Autodesk Fusion 360 part; units mm, degrees
sketch "Sketch1" plane through (0, 0, 0) normal (0, 1, 0) x (1, 0, 0) in component "Oil Drop Cap"
  circle A0 centre (0, 0) radius 6.2
  circle A1 centre (0, 0) radius 1.45
  dimension "d5" = 12.4
  dimension "d6" = 2.9
sketch "Sketch2" plane through (0, 0, 0) normal (1, 0, 0) x (0, 0, -1) in component "Oil Drop Cap"
  line L0 (0, 0) -> (0, 3.8) construction
  circle A0 centre (0, 3.8) radius 1.45
  dimension "d7" = 3.8
  dimension "d8" = 2.9
extrude "Extrude1" add sketch "Sketch1" along normal blind 10.3 contours A0 | A1 in component "Oil Drop Cap"
extrude "Extrude2" cut sketch "Sketch2" along normal up to surface end surface at (6.1923, 6.8667, 0.309) in component "Oil Drop Cap"
extrude "Extrude3" cut sketch "Sketch1" along normal up to surface contours A1 end surface at (2.0667, 5.25, 0) in component "Oil Drop Cap"
chamfer "Chamfer1" distance 0.25 angle 45 2 faces at (1.6068, 10.3, -0.7965) (4.5882, 0, 0.3801) in component "Oil Drop Cap"
chamfer "Chamfer1" distance 0.25 angle 45 1 edges at (6.0281, 3.8, 1.45) in component "Oil Drop Cap"
component "Oil Drop Cap" placed x (1, 0, 0) y (0, 1, 0) z (0, 0, 1) at (0, 0, 0)
equation "CylinderDiameter = 12.4 mm"
equation "CylinderHeight = 10.3 mm"
equation "HoleDiameter = 2.9 mm"
equation "HoleHeight = 3.8 mm"
equation "d5 = CylinderDiameter"
equation "d6 = HoleDiameter"
equation "d7 = HoleHeight"
equation "d8 = HoleDiameter"
equation "d9 = CylinderHeight"
CAD build for the part. Positions are in the model's coordinates, mm. A direction names the side the tool comes from. Round coordinates to 2 decimals unless told otherwise and drop trailing zeros. Order: outer loops, then holes, each group sorted by start corner. A loop starts at its lowest first (then second) coordinate and runs counter-clockwise, first axis right, second up. Notation, with made-up numbers: (-39, 76.25) - (-18, 76.25) arc R20 cw to (-18, 82.25) - close; hole circle Ø8 at (-17.5, 17). An arc over 180 degrees is marked (long way). Answer as CSV lines item,"result". Start each with the question number.
1. Pin check, flat tips, straight feed: pin 1 (2.5 mm diameter, centred on x = 0, z = 0, fed in from -Y); pin 2 (5 mm diameter, centred on y = 4, z = 2.5, fed in from +X); pin 3 (1 mm diameter, centred on y = 4, z = -1.5, fed in from -X). Stop position of each tip, or through.
2. Pull direction Z, two halves, no side cores. Call faces 1 (the face through (-0.57, 2.35, -0.03)), 2 (the face through (0, 10.3, 0)), 3 (the face through (2.86, 5.08, -5.5)): +Z half, -Z half, draft (parallel to the pull), parting line (faces both ways), or undercut.
3. Saw through at A-A, the plane y = 9. Write the cut outline in (x, z).
4. Tool access for faces 4 (the face through (2.933, 5.216, 0.314)), 5 (the face through (1.24, 0, -1.41)), 6 (the face through (0, 4, 0)): list every direction of +Z, -Z, +X, -X, +Y, -Y with a clear straight run to the whole face (end or side of a thin tool).
5. Drill centre lines: L1, parallel to Y at x = 3, z = 0; L2, parallel to X at y = 1.3, z = 0; L3, parallel to Z at x = -1.75, y = 3.25. Where is each one in solid material? Low to high. Write a range as [from, to].
Model answer:
1,pin 1,"stops at y = 2.35"
1,pin 2,"stops at x = 6.18"
1,pin 3,"stops at x = -6.12"
2,face 1,"undercut"
2,face 2,"draft"
2,face 3,"parting line"
3,outline,"circle Ø12.4 at (0, 0)"
4,face 4,"+X"
4,face 5,"+Z, -Z, +X, -X, -Y"
4,face 6,"+X, -Y"
5,L1,"y = [0, 2.35], [5.25, 10.3]"
5,L2,"x = [-6.2, -1.45], [1.45, 6.2]"
5,L3,"z = [-5.95, 5.95]"
